```python
from build123d import *

# Parameters (mm, degrees)
F_3_5_3_5_DIAMETER_HOLE1_D     = 3.5
F_3_5_3_5_DIAMETER_HOLE1_DEPTH = 5


with BuildPart() as part:
    # Sketch2 → Revolve1 (revolve)
    with BuildSketch(Plane.XZ, mode=Mode.PRIVATE) as revolve1_sk:
        Polygon((18, 30), (0, 30), (0, -17), (4, -17), (4, 0), (18, 0), align=None)
    revolve(revolve1_sk.sketch.rotate(Axis((0, 0, 30), (0, 0, -1)), 180), axis=Axis((0, 0, 30), (0, 0, -1)))

    # Ø3.5 (3.5) Diameter Hole1
    with Locations(Plane(origin=(0, 0, 0), x_dir=(-1, 0, 0), z_dir=(0, 0, -1))):
        with Locations((9.899494937, 9.899494937), (-9.899494937, -9.899494937), (9.899494937, -9.899494937), (-9.899494937, 9.899494937)):
            Hole(F_3_5_3_5_DIAMETER_HOLE1_D / 2, depth=F_3_5_3_5_DIAMETER_HOLE1_DEPTH)


solid = part.part
```
Here's how the part is built. I have some questions about the finished solid (model axes, mm). A direction names the side the tool comes from. Give positions to 0.01 mm unless a question says otherwise; leave off trailing zeros. Order: outer loops, then holes, each group sorted by start corner. A loop starts at its lowest first (then second) coordinate and runs counter-clockwise, first axis right, second up. Notation, with made-up numbers: (64, -17) - (116, -17) arc R32 ccw to (116, 18) - close; hole circle Ø1 at (54, 85.5). An arc over 180 degrees is marked (long way). Answer as a JSON object with one key per item and string values. Group by question number.
Item 1: If we mould it in two halves opening along Y, with no side actions, what happens to faces 3 (the flat face through (-4.3, 0.3, 0)), 4 (the cylindrical face through (8.15, 9.98, 2.54)), 5 (the cylindrical face through (13.267, 12.165, 15.21))? For each: pulls with the +Y half, pulls with the -Y half, needs draft (parallel to the pull), parting line crosses it, or undercut.
Item 2: For P1, Ø1, axis at x = -9, y = 9.5, coming from the -Z side; P2, Ø3, axis at x = 9.5, y = 10.5, coming from the -Z side; P3, Ø6, axis at y = -4, z = -10.5, coming from the +X side, each with a flat end and sliding along its axis, tell me the tip position at first contact or that it passes through.
Item 3: If we section it at D-D on y = -10.5: Please give me the cut outline in (x, z), and give its area (3 significant figures).
Item 4: Please list where these lines run through material, in increasing order: probe 1 along Z at (x, y) = (11, 1.5); probe 2 along Z at (x, y) = (9, -9.5); probe 3 along X at (y, z) = (-0.5, 11).
Item 5: Which directions (+Z, -Z, +X, -X, +Y, -Y) give clear straight access to the entire face, cutting with the end or side of a thin tool? Please do faces 1 (the flat face through (10, 10, 5)), 2 (the flat face through (0, 0, -17)).
Item 6: If we section it at A-A on x = 0: Please give me the cut outline in (y, z), and give its area (3 significant figures).
Item 7: If we section it at C-C on z = -4: Please give me the cut outline in (x, y).
Result set:
{
 "1": {"face 3": "needs draft", "face 4": "undercut", "face 5": "parting line crosses it"},
 "2": {"P1": "z = 5", "P2": "z = 0", "P3": "x = 3.87"},
 "3": {"outline": "(-14.62, 0) - (-11.54, 0) - (-11.54, 5) - (-8.26, 5) - (-8.26, 0) - (8.26, 0) - (8.26, 5) - (11.54, 5) - (11.54, 0) - (14.62, 0) - (14.62, 30) - (-14.62, 30) - close", "area": "844 mm²"},
 "4": {"probe 1": "0 to 30", "probe 2": "5 to 30", "probe 3": "-17.99 to 17.99"},
 "5": {"face 1": "-Z", "face 2": "-Z, +X, -X, +Y, -Y"},
 "6": {"outline": "(-18, 0) - (-4, 0) - (-4, -17) - (4, -17) - (4, 0) - (18, 0) - (18, 30) - (-18, 30) - close", "area": "1,220 mm²"},
 "7": {"outline": "circle Ø8 at (0, 0)"}
}
